```python
from build123d import *

# Parameters (mm, degrees)
EXTRUDE_1_DEPTH       = 30
EXTRUDE_8_DEPTH       = 30
SKETCH_2_W            = 6.2
SKETCH_2_H            = 6.2
CUT_EXTRUDE_5_DEPTH   = 1
EXTRUDE_9_DEPTH       = 6.2
EXTRUDE_9_DEPTH_BACK  = 23.8
SKETCH_15_W           = 6.2
SKETCH_15_H           = 6.2
CUT_EXTRUDE_10_DEPTH  = 1
EXTRUDE_10_DEPTH      = 6.2
EXTRUDE_10_DEPTH_BACK = 23.8
EXTRUDE_11_DEPTH      = 6.2
EXTRUDE_11_DEPTH_BACK = 23.8
SKETCH_20_W           = 6.2
SKETCH_20_H           = 6.2
CUT_EXTRUDE_11_DEPTH  = 1
EXTRUDE_12_DEPTH      = 6.2
EXTRUDE_12_DEPTH_BACK = 23.8
EXTRUDE_13_DEPTH      = 6.2
EXTRUDE_13_DEPTH_BACK = 23.8
EXTRUDE_14_DEPTH      = 6.2
EXTRUDE_14_DEPTH_BACK = 23.8
SKETCH_25_R           = 5
EXTRUDE_15_DEPTH      = 10


with BuildPart() as part:
    # ｽｹｯﾁ1 → ﾎﾞｽ - 押し出し1 (new body)
    with BuildSketch(Plane.XY):
        Polygon((0, 21.650635095), (-12.5, 0), (12.5, 0), align=None)
    extrude(amount=EXTRUDE_1_DEPTH)

    # ｽｹｯﾁ11 → ﾎﾞｽ - 押し出し8 (add, through all)
    with BuildSketch(Plane(origin=(0, 0, 0), x_dir=(-1, 0, 0), z_dir=(0, 0, -1))):
        with BuildLine():
            Line((0.866025404, 22.150635095), (13.366025404, 0.5))
            ThreePointArc((13.366025404, 0.5), (13.243672874, -0.429359734), (12.5, -1))
            Line((12.5, -1), (-12.5, -1))
            ThreePointArc((-12.5, -1), (-13.243672874, -0.429359734), (-13.366025404, 0.5))
            Line((-13.366025404, 0.5), (-0.866025404, 22.150635095))
            ThreePointArc((-0.866025404, 22.150635095), (0, 22.509354562), (0.866025404, 22.150635095))
        make_face()
        Polygon((0, 21.650635095), (12.5, 0), (-12.5, 0), align=None, mode=Mode.SUBTRACT)
    extrude(amount=-EXTRUDE_8_DEPTH)

    # ｽｹｯﾁ2 → ｶｯﾄ - 押し出し5 (cut)
    with BuildSketch(Plane(origin=(-9.375, 5.412658774, 0), x_dir=(0, 0, 1), z_dir=(-0.866025404, 0.5, 0))):
        with Locations((26.9, -3.15)):
            Rectangle(SKETCH_2_W, SKETCH_2_H)
        with Locations((26.9, 15.65)):
            Rectangle(SKETCH_2_W, SKETCH_2_H)
        with Locations((8.1, -3.15)):
            Rectangle(SKETCH_2_W, SKETCH_2_H)
        with Locations((8.1, 15.65)):
            Rectangle(SKETCH_2_W, SKETCH_2_H)
    extrude(amount=CUT_EXTRUDE_5_DEPTH, mode=Mode.SUBTRACT)

    # ｽｹｯﾁ16 → ﾎﾞｽ - 押し出し9 (add, two sides)
    with BuildSketch(Plane.XY.offset(23.8)) as extrude_9_sk:
        Polygon((-12.4, 0.173205081), (-12.673205081, 0.1), (-12.5, 0), align=None)
    extrude(amount=EXTRUDE_9_DEPTH)
    extrude(extrude_9_sk.sketch, amount=-EXTRUDE_9_DEPTH_BACK)

    # ｽｹｯﾁ15 → ｶｯﾄ - 押し出し10 (cut)
    with BuildSketch(Plane.XZ):
        with Locations((-9.4, 26.9)):
            Rectangle(SKETCH_15_W, SKETCH_15_H)
        with Locations((9.4, 26.9)):
            Rectangle(SKETCH_15_W, SKETCH_15_H)
        with Locations((9.4, 8.1)):
            Rectangle(SKETCH_15_W, SKETCH_15_H)
        with Locations((-9.4, 8.1)):
            Rectangle(SKETCH_15_W, SKETCH_15_H)
    extrude(amount=CUT_EXTRUDE_10_DEPTH, mode=Mode.SUBTRACT)

    # ｽｹｯﾁ18 → ﾎﾞｽ - 押し出し10 (add, two sides)
    with BuildSketch(Plane.XY.offset(23.8)) as extrude_10_sk:
        Polygon((-0.173205081, 21.750635095), (0, 21.650635095), (-0.1, 21.477430014), align=None)
    extrude(amount=EXTRUDE_10_DEPTH)
    extrude(extrude_10_sk.sketch, amount=-EXTRUDE_10_DEPTH_BACK)

    # ｽｹｯﾁ19 → ﾎﾞｽ - 押し出し11 (add, two sides)
    with BuildSketch(Plane.XY.offset(23.8)) as extrude_11_sk:
        Polygon((12.5, 0), (12.3, 0), (12.5, -0.2), align=None)
    extrude(amount=EXTRUDE_11_DEPTH)
    extrude(extrude_11_sk.sketch, amount=-EXTRUDE_11_DEPTH_BACK)

    # ｽｹｯﾁ20 → ｶｯﾄ - 押し出し11 (cut)
    with BuildSketch(Plane(origin=(9.375, 5.412658774, 0), x_dir=(0, 0, -1), z_dir=(0.866025404, 0.5, 0))):
        with Locations((-26.9, -3.15)):
            Rectangle(SKETCH_20_W, SKETCH_20_H)
        with Locations((-26.9, 15.65)):
            Rectangle(SKETCH_20_W, SKETCH_20_H)
        with Locations((-8.1, -3.15)):
            Rectangle(SKETCH_20_W, SKETCH_20_H)
        with Locations((-8.1, 15.65)):
            Rectangle(SKETCH_20_W, SKETCH_20_H)
    extrude(amount=CUT_EXTRUDE_11_DEPTH, mode=Mode.SUBTRACT)

    # ｽｹｯﾁ21 → ﾎﾞｽ - 押し出し12 (add, two sides)
    with BuildSketch(Plane.XY.offset(23.8)) as extrude_12_sk:
        Polygon((0, 21.650635095), (0.1, 21.477430014), (0.173205081, 21.750635095), align=None)
    extrude(amount=EXTRUDE_12_DEPTH)
    extrude(extrude_12_sk.sketch, amount=-EXTRUDE_12_DEPTH_BACK)

    # ｽｹｯﾁ23 → ﾎﾞｽ - 押し出し13 (add, two sides)
    with BuildSketch(Plane.XY.offset(23.8)) as extrude_13_sk:
        Polygon((12.5, 0), (12.673205081, 0.1), (12.4, 0.173205081), align=None)
    extrude(amount=EXTRUDE_13_DEPTH)
    extrude(extrude_13_sk.sketch, amount=-EXTRUDE_13_DEPTH_BACK)

    # ｽｹｯﾁ24 → ﾎﾞｽ - 押し出し14 (add, two sides)
    with BuildSketch(Plane.XY.offset(23.8)) as extrude_14_sk:
        Polygon((-12.5, 0), (-12.3, 0), (-12.5, -0.2), align=None)
    extrude(amount=EXTRUDE_14_DEPTH)
    extrude(extrude_14_sk.sketch, amount=-EXTRUDE_14_DEPTH_BACK)

    # ｽｹｯﾁ25 → ﾎﾞｽ - 押し出し15 (add)
    with BuildSketch(Plane(origin=(0, 0, 0), x_dir=(-1, 0, 0), z_dir=(0, 0, -1))):
        with Locations((0, 7.216878365)):
            Circle(SKETCH_25_R)
    extrude(amount=EXTRUDE_15_DEPTH)


solid = part.part
```
Work out the finished part from the listing and answer in its coordinate system (mm). A direction names the side the tool comes from. Give positions to 0.01 mm unless a question says otherwise; leave off trailing zeros. Loops run counter-clockwise (first coordinate to the right, second up) from the corner with the lowest first, then second, coordinate; pieces in that order, holes last. Notation, with made-up numbers: (67, 23) - (80, 23) arc R29 cw to (80, 45) - close; hole circle Ø2 at (40.25, 59.5). An arc over 180 degrees is marked (long way). One line per question, with ' | ' between items.
(1) The mould has two halves that part along Y. Classify faces 1 (the face through (-13.25, -0.42, 14.79)), 2 (the face through (7.204, 11.174, 14.79)), 3 (the face through (-1.579, 18.916, 26.857)): +Y half, -Y half, draft (parallel to the pull), parting line (faces both ways), or undercut.
Recorded:
face 1: parting line | face 2: +Y half | face 3: undercut
(2) The part is cut by section D-D (y = 8.75). Write down the section's boundary in (x, z).
Recorded:
outline: (-8.6, 0) - (-4.76, 0) - (-4.76, -10) - (4.76, -10) - (4.76, 0) - (8.6, 0) - (8.6, 30) - (-8.6, 30) - close
(3) The part is cut by section B-B (y = 3). Write down the section's boundary in (x, z).
Recorded:
outline: (-11.92, 0) - (-2.69, 0) - (-2.69, -10) - (2.69, -10) - (2.69, 0) - (11.92, 0) - (11.92, 5) - (10.77, 5) - (10.77, 11.2) - (11.92, 11.2) - (11.92, 23.8) - (10.77, 23.8) - (10.77, 30) - (-10.77, 30) - (-10.77, 23.8) - (-11.92, 23.8) - (-11.92, 11.2) - (-10.77, 11.2) - (-10.77, 5) - (-11.92, 5) - close
(4) Straight lines are drawn through the part: probe 1 along Z at (x, y) = (-1.5, 1); probe 2 along Y at (x, z) = (10, 27.5); probe 3 along X at (y, z) = (21.5, 24). For each, find the intervals that lie inside material, in ascending order.
Recorded:
probe 1: z = 0 to 30 | probe 2: y = 0 to 4.33, 5.72 to 6.33 | probe 3: x = -0.11 to 0.11
(5) The part is cut by section A-A (z = 12). Write down the section's boundary in (x, y), then the cut area to 3 significant figures.
Recorded:
outline: (-13.37, 0.5) arc R1.22 ccw to (-12.5, -1) - (12.5, -1) arc R1.22 ccw to (13.37, 0.5) - (0.87, 22.15) arc R1.22 ccw to (-0.87, 22.15) - close | area: 348 mm²
(6) A tool of negligible diameter and unlimited length cuts with its end or side. For faces 4 (the face through (9.8, 5.6, 8.1)), 5 (the face through (-3.53, 16.53, 8.06)), 6 (the face through (3.53, 16.53, 26.94)), 7 (the face through (9, 0, 27)), 8 (the face through (6.3, -0.5, 8.1)), from which of +Z, -Z, +X, -X, +Y, -Y can it reach the whole face along a straight path? Write none if from no direction.
Recorded:
face 4: +X | face 5: +Y | face 6: +Z, +Y | face 7: +Z, -Y | face 8: -Y
(7) The part is cut by section C-C (x = 8). Write down the section's boundary in (y, z), then the cut area to 3 significant figures.
Recorded:
outline: (-1, 0) - (9.79, 0) - (9.79, 30) - (0, 30) - (0, 23.8) - (-1, 23.8) - (-1, 11.2) - (0, 11.2) - (0, 5) - (-1, 5) - close | area: 311 mm²
(8) Each of these flat-tipped pins is pushed along its axis until it touches: pin 1 Ø0.8 at (y, z) = (-0.5, 7.5) entering from +X; pin 2 Ø1.8 at (x, z) = (8, 28.5) entering from -Y; pin 3 Ø1.5 at (y, z) = (12.5, 4) entering from +X; pin 4 Ø1.2 at (x, y) = (1, 20) entering from +Z. Where does it stop, or does it pass through?
Recorded:
pin 1: stops at x = 13.37 | pin 2: stops at y = 0 | pin 3: stops at x = 6.87 | pin 4: stops at z = 30
